from build123d import *

# Parameters (mm, degrees)
SKETCH1_W                           = 198.43248
SKETCH1_H                           = 59.281
SKETCH1_R                           = 1.5
BOSS_EXTRUDE1_DEPTH                 = 4.5
SKETCH4_W                           = 9.531640124
SKETCH4_H                           = 18.749999962
SKETCH4_W_2                         = 9.531640123
CUT_EXTRUDE2_DEPTH                  = 149.263073085
CUT_EXTRUDE3_DEPTH                  = 149.263073085
SKETCH6_W                           = 198.43248
SKETCH6_H                           = 4.22
BOSS_EXTRUDE2_DEPTH                 = 4.5
CUT_EXTRUDE4_DEPTH                  = 152.422689452
FILLET1_R                           = 7.62
F_27_0_144_DIAMETER_SLOT1_OUTLINE_R = 1.5
F_27_0_144_DIAMETER_SLOT1_DEPTH     = 4.5


# Read off the part's stored shape, not the designer's step: #27 (0.144) Diameter Slot1
with BuildPart() as part:
    # Sketch1 → Boss-Extrude1 (new body)
    with BuildSketch(Plane.XY):
        with Locations((0, 80.4405)):
            Rectangle(SKETCH1_W, SKETCH1_H)
        with Locations((46.2, 105.081)):
            Circle(SKETCH1_R, mode=Mode.SUBTRACT)
        with Locations((46.2, 65.8)):
            Circle(SKETCH1_R, mode=Mode.SUBTRACT)
        with Locations((15.4, 65.8)):
            Circle(SKETCH1_R, mode=Mode.SUBTRACT)
        with Locations((15.4, 105.081)):
            Circle(SKETCH1_R, mode=Mode.SUBTRACT)
        with Locations((-15.4, 105.081)):
            Circle(SKETCH1_R, mode=Mode.SUBTRACT)
        with Locations((-15.4, 65.8)):
            Circle(SKETCH1_R, mode=Mode.SUBTRACT)
    extrude(amount=BOSS_EXTRUDE1_DEPTH)

    # Sketch4 → Cut-Extrude2 (cut, through all)
    with BuildSketch(Plane(origin=(0, 0, 4.5), x_dir=(-1, 0, 0), z_dir=(0, 0, -1))):
        with Locations((-53.889258182, 90.503714938)):
            Rectangle(SKETCH4_W, SKETCH4_H)
        with Locations((-38.492327273, 90.503714938)):
            Rectangle(SKETCH4_W, SKETCH4_H)
        with Locations((-23.095396364, 90.503714938)):
            Rectangle(SKETCH4_W_2, SKETCH4_H)
        with Locations((-7.698465454, 90.503714938)):
            Rectangle(SKETCH4_W_2, SKETCH4_H)
        with Locations((7.698465454, 90.503714938)):
            Rectangle(SKETCH4_W_2, SKETCH4_H)
        with Locations((23.095396364, 90.503714938)):
            Rectangle(SKETCH4_W_2, SKETCH4_H)
    extrude(amount=CUT_EXTRUDE2_DEPTH, mode=Mode.SUBTRACT)

    # Sketch5 → Cut-Extrude3 (cut, through all)
    with BuildSketch(Plane(origin=(0, 0, 0), x_dir=(-1, 0, 0), z_dir=(0, 0, -1))):
        with BuildLine():
            Line((-74.899953, 69.8), (-74.899953, 61.8))
            ThreePointArc((-74.899953, 61.8), (-76.999953, 59.7), (-79.099953, 61.8))
            Line((-79.099953, 61.8), (-79.099953, 69.8))
            ThreePointArc((-79.099953, 69.8), (-76.999953, 71.9), (-74.899953, 69.8))
        make_face()
        with BuildLine():
            Line((44.099953, 69.8), (44.099953, 61.8))
            ThreePointArc((44.099953, 61.8), (46.199953, 59.7), (48.299953, 61.8))
            Line((48.299953, 61.8), (48.299953, 69.8))
            ThreePointArc((48.299953, 69.8), (46.199953, 71.9), (44.099953, 69.8))
        make_face()
    extrude(amount=-CUT_EXTRUDE3_DEPTH, mode=Mode.SUBTRACT)

    # Sketch6 → Boss-Extrude2 (add)
    with BuildSketch(Plane(origin=(0, 0, 0), x_dir=(-1, 0, 0), z_dir=(0, 0, -1))):
        with Locations((0, 112.191)):
            Rectangle(SKETCH6_W, SKETCH6_H)
    extrude(amount=-BOSS_EXTRUDE2_DEPTH)

    # Sketch7 → Cut-Extrude4 (cut, through all)
    with BuildSketch(Plane(origin=(0, 0, 0), x_dir=(-1, 0, 0), z_dir=(0, 0, -1))):
        Polygon((-68.815078244, 114.301), (-99.21624, 114.301), (-99.21624, 50.8), (-95.088898012, 50.8), (-84.050148524, 81.128714957), (-68.815078244, 81.128714957), align=None)
        Polygon((99.21624, 114.301), (38.015078244, 114.301), (38.015078244, 81.128714957), (53.250148524, 81.128714957), (64.288898012, 50.8), (99.21624, 50.8), align=None)
    extrude(amount=-CUT_EXTRUDE4_DEPTH, mode=Mode.SUBTRACT)

    # Fillet1
    fillet1_edges = [part.edges().sort_by_distance(p)[0] for p in [
        (84.050148524, 81.128714957, 2.25),
        (68.815078244, 81.128714957, 2.25),
        (-53.250148524, 81.128714957, 2.25),
        (-38.015078244, 81.128714957, 2.25),
    ]]
    fillet(fillet1_edges, radius=FILLET1_R)

    # #27 (0.144) Diameter Slot1 outline → #27 (0.144) Diameter Slot1 (cut)
    # profile 1 of 6: a face of its own
    with BuildSketch(Plane.XY):
        with BuildLine():
            ThreePointArc((49.4512, 103.2522), (51.28, 105.081), (49.4512, 106.9098))
            Line((49.4512, 106.9098), (42.9488, 106.9098))
            ThreePointArc((42.9488, 106.9098), (41.12, 105.081), (42.9488, 103.2522))
            Line((42.9488, 103.2522), (49.4512, 103.2522))
        make_face()
        with Locations((46.2, 105.081)):
            Circle(F_27_0_144_DIAMETER_SLOT1_OUTLINE_R, mode=Mode.SUBTRACT)
    # profile 2 of 6: a face of its own
    with BuildSketch(Plane.XY):
        with BuildLine():
            ThreePointArc((12.1488, 106.9098), (10.32, 105.081), (12.1488, 103.2522))
            Line((12.1488, 103.2522), (18.6512, 103.2522))
            ThreePointArc((18.6512, 103.2522), (20.48, 105.081), (18.6512, 106.9098))
            Line((18.6512, 106.9098), (12.1488, 106.9098))
        make_face()
        with Locations((15.4, 105.081)):
            Circle(F_27_0_144_DIAMETER_SLOT1_OUTLINE_R, mode=Mode.SUBTRACT)
    # profile 3 of 6: a face of its own
    with BuildSketch(Plane.XY):
        with BuildLine():
            ThreePointArc((-18.6512, 106.9098), (-20.48, 105.081), (-18.6512, 103.2522))
            Line((-18.6512, 103.2522), (-12.1488, 103.2522))
            ThreePointArc((-12.1488, 103.2522), (-10.32, 105.081), (-12.1488, 106.9098))
            Line((-12.1488, 106.9098), (-18.6512, 106.9098))
        make_face()
        with Locations((-15.4, 105.081)):
            Circle(F_27_0_144_DIAMETER_SLOT1_OUTLINE_R, mode=Mode.SUBTRACT)
    # profile 4 of 6: a face of its own
    with BuildSketch(Plane.XY):
        with BuildLine():
            ThreePointArc((-12.1488, 63.9712), (-10.32, 65.8), (-12.1488, 67.6288))
            Line((-12.1488, 67.6288), (-18.6512, 67.6288))
            ThreePointArc((-18.6512, 67.6288), (-20.48, 65.8), (-18.6512, 63.9712))
            Line((-18.6512, 63.9712), (-12.1488, 63.9712))
        make_face()
        with Locations((-15.4, 65.8)):
            Circle(F_27_0_144_DIAMETER_SLOT1_OUTLINE_R, mode=Mode.SUBTRACT)
    # profile 5 of 6: a face of its own
    with BuildSketch(Plane.XY):
        with BuildLine():
            ThreePointArc((12.1488, 67.6288), (10.32, 65.8), (12.1488, 63.9712))
            Line((12.1488, 63.9712), (18.6512, 63.9712))
            ThreePointArc((18.6512, 63.9712), (20.48, 65.8), (18.6512, 67.6288))
            Line((18.6512, 67.6288), (12.1488, 67.6288))
        make_face()
        with Locations((15.4, 65.8)):
            Circle(F_27_0_144_DIAMETER_SLOT1_OUTLINE_R, mode=Mode.SUBTRACT)
    # profile 6 of 6: a face of its own
    with BuildSketch(Plane.XY):
        with BuildLine():
            ThreePointArc((42.9488, 67.6288), (41.12, 65.8), (42.9488, 63.9712))
            Line((42.9488, 63.9712), (49.4512, 63.9712))
            ThreePointArc((49.4512, 63.9712), (51.28, 65.8), (49.4512, 67.6288))
            Line((49.4512, 67.6288), (42.9488, 67.6288))
        make_face()
        with Locations((46.2, 65.8)):
            Circle(F_27_0_144_DIAMETER_SLOT1_OUTLINE_R, mode=Mode.SUBTRACT)
    extrude(amount=F_27_0_144_DIAMETER_SLOT1_DEPTH, mode=Mode.SUBTRACT)


solid = part.part
The model under review builds one solid part; all positions refer to its coordinate system, in mm. A direction names the side the tool comes from. Round coordinates to 2 decimals unless told otherwise and drop trailing zeros. Order: outer loops, then holes, each group sorted by start corner. A loop starts at its lowest first (then second) coordinate and runs counter-clockwise, first axis right, second up. Notation, with made-up numbers: (-6.5, -15.75) -> (50.5, -15.75) arc R22 ccw to (50.5, 10.25) -> close; hole circle Ø6 at (40, 42). An arc over 180 degrees is marked (long way). Write item = value, one per line. Start each with the question number.
Item 1: Consider section B-B on y = 65.8. Write out the cut boundary in (x, z).
Item 2: Consider section D-D on y = 55. Write out the cut boundary in (x, z), plus the area to 3 significant figures.
Item 3: Clearance check with flat-ended pins moving along their axes: pin 1 Ø0.7 at (x, z) = (-46.5, 2.5) entering from +Y; pin 2 Ø1.3 at (y, z) = (92.5, 1.5) entering from +X; pin 3 Ø1.3 at (y, z) = (92, 3) entering from -X. State where each tip first meets the part, or that it passes through.
Item 4: Consider section A-A on x = 25.5. Write out the cut boundary in (y, z).
Item 5: For line 1 along Y through (x, z) = (-9.5, 2.3); line 2 along Y through (x, z) = (50, 3.25); line 3 along X through (y, z) = (60.5, 0.65), list the stretches that pass through material, from the lowest coordinate up.
Item 6: Consider section C-C on z = 2.1. Count the separate pieces of the cut face and the enclosed holes in it, plus the area to 3 significant figures.
Item 7: Mouldability with a two-part tool opening along Y and no side actions: class faces 5 (the face through (17, 76, 0)), 6 (the face through (39, 81.129, 2)), 7 (the face through (-40.19, 83.42, 2.28)) as released by +Y, released by -Y, zero draft, split by the parting line, or undercut.
Item 8: For faces 1 (the face through (-38.015, 102, 2)), 2 (the face through (16, 114.301, 2)), 3 (the face through (68.815, 101, 2)), 4 (the face through (54, 81.129, 2)), list the 3-axis set-ups (+Z, -Z, +X, -X, +Y, -Y) from which the entire face can be reached by the end or side of a thin tool; tool diameter is ignored.
Conclusion:
q1.outline = (-58.83, 0) -> (-48.3, 0) -> (-48.3, 4.5) -> (-58.83, 4.5) -> close; (-44.1, 0) -> (-20.48, 0) -> (-20.48, 4.5) -> (-44.1, 4.5) -> close; (-10.32, 0) -> (10.32, 0) -> (10.32, 4.5) -> (-10.32, 4.5) -> close; (20.48, 0) -> (41.12, 0) -> (41.12, 4.5) -> (20.48, 4.5) -> close; (51.28, 0) -> (74.9, 0) -> (74.9, 4.5) -> (51.28, 4.5) -> close; (79.1, 0) -> (89.63, 0) -> (89.63, 4.5) -> (79.1, 4.5) -> close
q2.outline = (-62.76, 0) -> (93.56, 0) -> (93.56, 4.5) -> (-62.76, 4.5) -> close
q2.area = 703 mm2
q3.pin_1 = 81.13
q3.pin_2 = 68.82
q3.pin_3 = -38.02
q4.outline = (50.8, 0) -> (81.13, 0) -> (81.13, 4.5) -> (50.8, 4.5) -> close; (99.88, 0) -> (114.3, 0) -> (114.3, 4.5) -> (99.88, 4.5) -> close
q5.line_1 = 50.8 to 81.13, 99.88 to 114.3
q5.line_2 = 50.8 to 64.06, 67.54 to 81.13, 99.88 to 103.34, 106.83 to 114.3
q5.line_3 = -60.76 to -47.85, -44.55 to 75.35, 78.65 to 91.56
q6.separate_pieces = 1
q6.enclosed_holes = 14
q6.area = 6,680 mm2
q7.face_5 = zero draft
q7.face_6 = undercut
q7.face_7 = released by +Y
q8.face_1 = +Z, -Z, -X, +Y
q8.face_2 = +Z, -Z, +X, -X, +Y
q8.face_3 = +Z, -Z, +X, +Y
q8.face_4 = +Z, -Z
